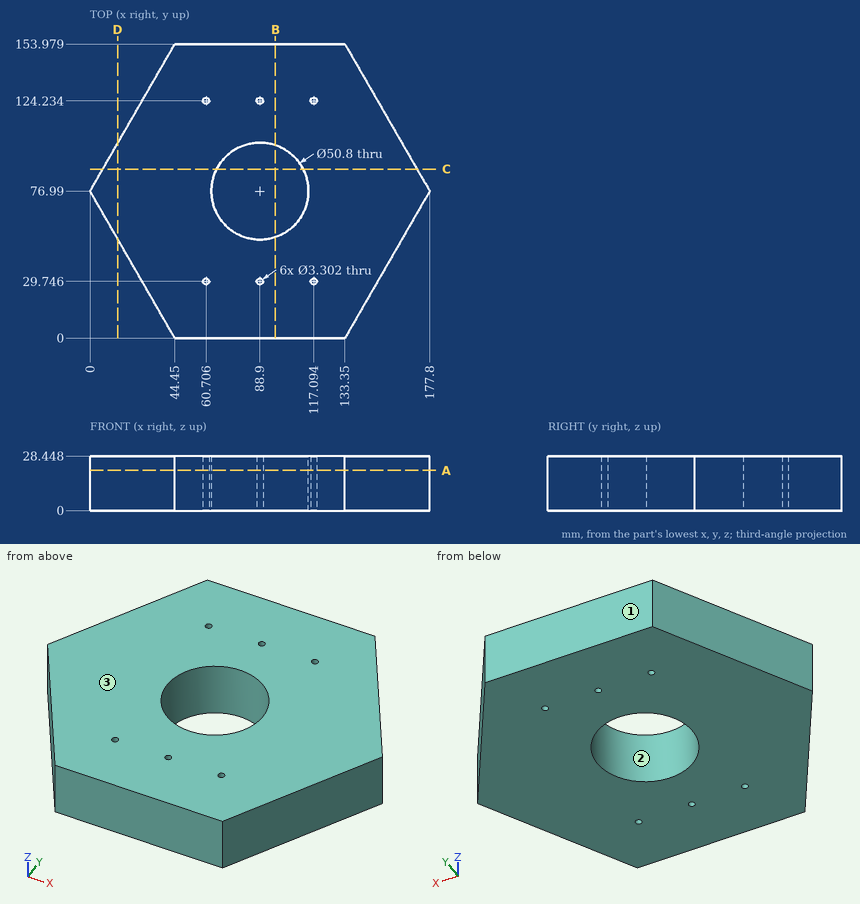
Answer from the drawing. Dimensions are ordinates in mm from the lowest x, y and z of the part. Round coordinates to 2 decimals unless told otherwise and drop trailing zeros. Loops run counter-clockwise (first coordinate to the right, second up) from the corner with the lowest first, then second, coordinate; pieces in that order, holes last. Notation, with made-up numbers: M 3,-9.75 L 14,-9.75 A12 ccw 14,12.25 Z; hole C -31,74.25 d5. An arc over 180 degrees is marked long. One line per question, with ' | ' between items. Start each with the question number.
(1) For a pull along Y with two mould halves and no side action, classify the marked faces 1, 2 and 3 as released by +Y, released by -Y, zero draft, split by the parting line, or undercut.
(2) A cutting plane is placed at A-A on z = 21. Give the number of separate pieces and of enclosed holes in the cut face, plus the area to 3 significant figures.
(3) A cutting plane is placed at C-C on y = 88.5. Write down the section's boundary in (x, z) (1 decimal).
(4) Flat-ended cylindrical pins translate along their axes: pin 1 Ø3 at (x, y) = (60.71, 124.23) entering from -Z; pin 2 Ø6 at (x, z) = (141, 23) entering from -Y (1 decimal); pin 3 Ø12 at (y, z) = (110.5, 10.5) entering from -X; pin 4 Ø2 at (y, z) = (132.5, 15.5) entering from -X. Find the tip coordinate at first contact, or state that the pin passes through.
(5) A cutting plane is placed at D-D on x = 14.5. Write down the section's boundary in (y, z) (1 decimal), plus the area to 3 significant figures.
(6) A cutting plane is placed at B-B on x = 97. Write down the section's boundary in (y, z).
(7) Find the intervals of material crossed by line 1 (Y direction, x = 88.9, z = 11) (1 decimal); line 2 (Y direction, x = 68, z = 3.25) (1 decimal); line 3 (Y direction, x = 116.5, z = 4.25) (1 decimal), in increasing order.
Geometry check:
1) face 1: released by +Y | face 2: undercut | face 3: zero draft
2) separate pieces: 1 | enclosed holes: 7 | area: 18,500 mm²
3) outline: M 6.6,0 L 66.3,0 L 66.3,28.4 L 6.6,28.4 Z; M 111.5,0 L 171.2,0 L 171.2,28.4 L 111.5,28.4 Z
4) pin 1: passes through | pin 2: stops at y = 8.1 | pin 3: stops at x = 15.88 | pin 4: stops at x = 31.47
5) outline: M 51.9,0 L 102.1,0 L 102.1,28.4 L 51.9,28.4 Z | area: 1,430 mm²
6) outline: M 0,0 L 52.92,0 L 52.92,28.45 L 0,28.45 Z; M 101.06,0 L 153.98,0 L 153.98,28.45 L 101.06,28.45 Z
7) line 1: y = 0 to 28.1, 31.4 to 51.6, 102.4 to 122.6, 125.9 to 154 | line 2: y = 0 to 62.6, 91.4 to 154 | line 3: y = 0 to 28.2, 31.3 to 122.7, 125.8 to 154
